Can you work these out from the model? Positions are in its coordinate system, mm. Give positions to 0.01 mm unless a question says otherwise; leave off trailing zeros. Order: outer loops, then holes, each group sorted by start corner. A loop starts at its lowest first (then second) coordinate and runs counter-clockwise, first axis right, second up. Notation, with made-up numbers: (-16.5, 39) - (16.5, 39) arc R23 cw to (16.5, 47) - close; hole circle Ø10 at (4, 39.5). An arc over 180 degrees is marked (long way). Use one line per item in the form item = value. Start each with the question number.
1) Please list where these lines run through material, in increasing order: probe 1 along Y at (x, z) = (9.5, 1.5); probe 2 along Y at (x, z) = (-0.5, 0.7); probe 3 along Y at (x, z) = (36, 1.5).
2) Suppose I cut it at B-B, the plane y = -10. Write out the boundary of the cut face in (x, z), and give its area (3 significant figures).
3) Suppose I cut it at D-D, the plane y = 10. Write out the boundary of the cut face in (x, z), and give its area (3 significant figures).
4) Suppose I cut it at A-A, the plane x = 9.5. Write out the boundary of the cut face in (y, z).
5) Suppose I cut it at C-C, the plane y = 0. Write out the boundary of the cut face in (x, z), and give its area (3 significant figures).
6) For pin 1 (0.6 mm diameter, centred on x = 15.5, z = 1.5, fed in from -Y); pin 2 (0.6 mm diameter, centred on y = -1.5, z = 0.5, fed in from +X); pin 3 (1 mm diameter, centred on y = 5.5, z = 1.5, fed in from +X), each with a flat end and sliding along its axis, tell me the tip position at first contact or that it passes through.
```python
from build123d import *

# Parameters (mm, degrees)
SKETCH_1_R      = 1.5
EXTRUDE_1_DEPTH = 2


with BuildPart() as part:
    # 草图1 → 凸台-拉伸1 (new body)
    with BuildSketch(Plane.XY):
        with BuildLine():
            Line((16.993865071, 16), (16.993865071, 20))
            Line((16.993865071, 20), (-15.993865071, 20))
            ThreePointArc((-15.993865071, 20), (-16.700971852, 19.707106781), (-16.993865071, 19))
            Line((-16.993865071, 19), (-16.993865071, 16))
            Line((-16.993865071, 16), (-19.993865071, 16))
            Line((-19.993865071, 16), (-19.993865071, 11))
            Line((-19.993865071, 11), (-16.993865071, 11))
            Line((-16.993865071, 11), (-16.993865071, 7.5))
            Line((-16.993865071, 7.5), (-14.493865071, 7.5))
            Line((-14.493865071, 7.5), (-14.493865071, 9))
            Line((-14.493865071, 9), (-11.893865071, 9))
            Line((-11.893865071, 9), (-11.893865071, 7.5))
            Line((-11.893865071, 7.5), (-8.893865071, 7.5))
            Line((-8.893865071, 7.5), (-8.893865071, 4.5))
            Line((-8.893865071, 4.5), (-11.893865071, 4.5))
            Line((-11.893865071, 4.5), (-11.893865071, 3))
            Line((-11.893865071, 3), (-14.493865071, 3))
            Line((-14.493865071, 3), (-14.493865071, 4.5))
            Line((-14.493865071, 4.5), (-16.993865071, 4.5))
            Line((-16.993865071, 4.5), (-16.993865071, 1))
            Line((-16.993865071, 1), (-19.993865071, 1))
            Line((-19.993865071, 1), (-19.993865071, -4))
            Line((-19.993865071, -4), (-16.993865071, -4))
            Line((-16.993865071, -4), (-16.993865071, -13))
            Line((-16.993865071, -13), (-16.993865071, -14))
            Line((-16.993865071, -14), (-0.721190694, -14))
            Line((-0.721190694, -14), (0, -15.5))
            Line((0, -15.5), (0.721190694, -14))
            Line((0.721190694, -14), (16.993865071, -14))
            Line((16.993865071, -14), (16.993865071, -13))
            Line((16.993865071, -13), (16.993865071, -4))
            Line((16.993865071, -4), (19.993865071, -4))
            Line((19.993865071, -4), (19.993865071, 1))
            Line((19.993865071, 1), (16.993865071, 1))
            Line((16.993865071, 1), (16.993865071, 4.5))
            Line((16.993865071, 4.5), (14.493865071, 4.5))
            Line((14.493865071, 4.5), (14.493865071, 3))
            Line((14.493865071, 3), (11.893865071, 3))
            Line((11.893865071, 3), (11.893865071, 4.5))
            Line((11.893865071, 4.5), (8.893865071, 4.5))
            Line((8.893865071, 4.5), (8.893865071, 7.5))
            Line((8.893865071, 7.5), (11.893865071, 7.5))
            Line((11.893865071, 7.5), (11.893865071, 9))
            Line((11.893865071, 9), (14.493865071, 9))
            Line((14.493865071, 9), (14.493865071, 7.5))
            Line((14.493865071, 7.5), (16.993865071, 7.5))
            Line((16.993865071, 7.5), (16.993865071, 11))
            Line((16.993865071, 11), (38.993865071, 11))
            Line((38.993865071, 11), (38.993865071, 16))
            Line((38.993865071, 16), (16.993865071, 16))
        make_face()
        with Locations((0, -10)):
            Circle(SKETCH_1_R, mode=Mode.SUBTRACT)
        Circle(SKETCH_1_R, mode=Mode.SUBTRACT)
        with Locations((0, 10)):
            Circle(SKETCH_1_R, mode=Mode.SUBTRACT)
        with BuildLine():
            Line((13.9, -11.15), (8.6, -11.15))
            ThreePointArc((8.6, -11.15), (8.123654403, -10), (8.6, -8.85))
            Line((8.6, -8.85), (13.9, -8.85))
            Line((13.9, -8.85), (13.9, -11.15))
        make_face(mode=Mode.SUBTRACT)
        with BuildLine():
            Line((-13.9, -8.85), (-8.6, -8.85))
            ThreePointArc((-8.6, -8.85), (-8.123654403, -10), (-8.6, -11.15))
            Line((-8.6, -11.15), (-13.9, -11.15))
            Line((-13.9, -11.15), (-13.9, -8.85))
        make_face(mode=Mode.SUBTRACT)
    extrude(amount=EXTRUDE_1_DEPTH)


solid = part.part
```
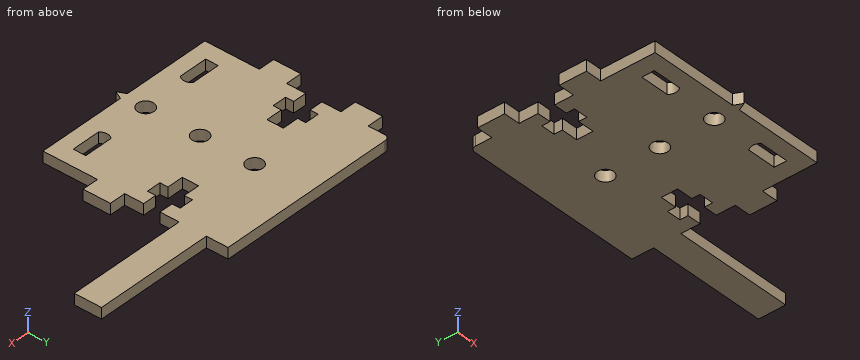
Result sheet:
q1.probe_1 = -14 to -11.15, -8.85 to 4.5, 7.5 to 20
q1.probe_2 = -14.46 to -11.41, -8.59 to -1.41, 1.41 to 8.59, 11.41 to 20
q1.probe_3 = 11 to 16
q2.outline = (-16.99, 0) - (-13.9, 0) - (-13.9, 2) - (-16.99, 2) - close; (-8.12, 0) - (-1.5, 0) - (-1.5, 2) - (-8.12, 2) - close; (1.5, 0) - (8.12, 0) - (8.12, 2) - (1.5, 2) - close; (13.9, 0) - (16.99, 0) - (16.99, 2) - (13.9, 2) - close
q2.area = 38.9 mm²
q3.outline = (-16.99, 0) - (-1.5, 0) - (-1.5, 2) - (-16.99, 2) - close; (1.5, 0) - (16.99, 0) - (16.99, 2) - (1.5, 2) - close
q3.area = 62.0 mm²
q4.outline = (-14, 0) - (-11.15, 0) - (-11.15, 2) - (-14, 2) - close; (-8.85, 0) - (4.5, 0) - (4.5, 2) - (-8.85, 2) - close; (7.5, 0) - (20, 0) - (20, 2) - (7.5, 2) - close
q5.outline = (-19.99, 0) - (-1.5, 0) - (-1.5, 2) - (-19.99, 2) - close; (1.5, 0) - (19.99, 0) - (19.99, 2) - (1.5, 2) - close
q5.area = 74.0 mm²
q6.pin_1 = -14
q6.pin_2 = 19.99
q6.pin_3 = 8.89
